```python
from build123d import *

# Parameters (mm, degrees)
BOSS_EXTRUDE1_DEPTH     = 31.75
F_1_4_CLEARANCE_HOLE1_D = 6.7564
CHAMFER1_SIZE           = 5.5
CHAMFER1_SIZE_2         = 31.192050008
CHAMFER2_SIZE           = 6
CHAMFER2_SIZE2          = 16.484864517


with BuildPart() as part:
    # Sketch1 → Boss-Extrude1 (new body)
    with BuildSketch(Plane.XY):
        Polygon((30.9, 0), (0, 0), (0, 29.5), (5.5, 29.5), (5.5, 4), (30.9, 4), align=None)
        Polygon((-44.5, 29.5), (0, 29.5), (5.5, 29.5), (5.5, 34.5), (-44.5, 34.5), align=None)
    extrude(amount=BOSS_EXTRUDE1_DEPTH)

    # 1/4 Clearance Hole1 (through all)
    with Locations(Plane(origin=(0, 4, 0), x_dir=(1, 0, 0), z_dir=(0, 1, 0))):
        with Locations((21.9, -23.495), (17.5, -8.255)):
            Hole(F_1_4_CLEARANCE_HOLE1_D / 2)

    # Chamfer1
    # the kernel refuses this chamfer: 31.192050008, 5.5 mm, written as the material it adds along each edge
    with BuildSketch(Plane(origin=(5.5, 4, 0), x_dir=(0.9776715712462578, -0.21013876076743532, 0), z_dir=(0, 0, 1))) as chamfer1_piece_1_section:
        Polygon((CHAMFER1_SIZE * 0.977671571246, CHAMFER1_SIZE * 0.210138760767), (-CHAMFER1_SIZE_2 * 0.210138760767, CHAMFER1_SIZE_2 * 0.977671571243), (0, 0), align=None)
    chamfer1_piece_1 = extrude(amount=31.75, mode=Mode.PRIVATE)
    chamfer1_piece_1 = split(chamfer1_piece_1, bisect_by=Plane(origin=(7.01069263, 34.5, 15.875), z_dir=(0, -1, 0)), keep=Keep.TOP, mode=Mode.PRIVATE)
    add(chamfer1_piece_1)

    # Chamfer2
    chamfer2_edges = [part.edges().sort_by_distance(p)[0] for p in [
        (0, 29.5, 15.875),
    ]]
    chamfer2_side = [part.faces().sort_by_distance(p)[0] for p in [
        (0, 14.75, 15.875),
    ]]
    chamfer(chamfer2_edges, length=CHAMFER2_SIZE, length2=CHAMFER2_SIZE2, reference=chamfer2_side[0])


solid = part.part
```
Input: part model. Units: mm. Frame: model coordinates. A direction names the side the tool comes from. Give positions to 0.01 mm unless a question says otherwise; leave off trailing zeros. Loops run counter-clockwise (first coordinate to the right, second up) from the corner with the lowest first, then second, coordinate; pieces in that order, holes last.
1) Section query B-B on z = 3. Return the cut outline in (x, y), and give its area (3 significant figures).
A:
outline: (-44.5, 29.5) - (-16.48, 29.5) - (0, 23.5) - (0, 0) - (30.9, 0) - (30.9, 4) - (11, 4) - (5.62, 34.5) - (-44.5, 34.5) - close
area: 649 mm2
2) Section query C-C on z = 24.5. Return the cut outline in (x, y).
A:
outline: (-44.5, 29.5) - (-16.48, 29.5) - (0, 23.5) - (0, 0) - (18.67, 0) - (18.67, 4) - (11, 4) - (5.62, 34.5) - (-44.5, 34.5) - close; (25.13, 0) - (30.9, 0) - (30.9, 4) - (25.13, 4) - close
3) Contact query for flat-ended pins moving along their axis: pin 1 (3 mm diameter, centred on x = -2, y = 19.5, fed in from -Z); pin 2 (6 mm diameter, centred on y = 17.5, z = 20.5, fed in from +X); pin 3 (12 mm diameter, centred on y = 12.5, z = 20, fed in from -X); pin 4 (8 mm diameter, centred on x = 17.5, z = 8.255, fed in from +Y). Output: stop coordinate, or through.
A:
pin 1: passes through
pin 2: stops at x = 9.15
pin 3: stops at x = 0
pin 4: stops at y = 4
4) Section query A-A on x = 17.5. Return the cut outline in (y, z), and give its area (4 significant figures).
A:
outline: (0, 0) - (4, 0) - (4, 4.88) - (0, 4.88) - close; (0, 11.63) - (4, 11.63) - (4, 31.75) - (0, 31.75) - close
area: 100.0 mm2
5) Section query D-D on x = -34. Return the cut outline in (y, z), and give its area (3 significant figures).
A:
outline: (29.5, 0) - (34.5, 0) - (34.5, 31.75) - (29.5, 31.75) - close
area: 159 mm2
6) Line query: L1, parallel to Z at x = 21.9, y = 0.85; L2, parallel to Y at x = 16, z = 16; L3, parallel to Y at x = -17, z = 21. Output: solid intervals per line, ascending.
A:
L1: z = 0 to 20.12, 26.87 to 31.75
L2: y = 0 to 4
L3: y = 29.5 to 34.5
7) Reachability of faces 1 (the flat face through (0, 12, 16)), 2 (the flat face through (-5, 26, 31.75)), 3 (the flat face through (21, 4, 16)) from +Z, -Z, +X, -X, +Y, -Y: full face, straight path, thin tool, end or side. Return the list, or none.
A:
face 1: +Z, -Z, -X, -Y
face 2: +Z, +X, -X, +Y, -Y
face 3: +Z, -Z, +X, +Y
8) Mould query, pull axis X, two halves, no side actions, for faces 4 (the cylindrical face through (14.278, 1.972, 7.24)), 5 (the flat face through (-19, 34.5, 16)), 6 (the flat face through (-44.5, 32, 16)). Classes: released by +X, released by -X, zero draft, split by the parting line, or undercut.
A:
face 4: undercut
face 5: zero draft
face 6: released by -X
